Verification items for the finished model (mm, model axes). A direction names the side the tool comes from. Coordinates: 2 decimals unless noted, no trailing zeros. Order: outer loops, then holes, each group sorted by start corner. A loop starts at its lowest first (then second) coordinate and runs counter-clockwise, first axis right, second up. Notation, with made-up numbers: M 1.25,43.25 L 32.25,43.25 A21 cw 32.25,63.25 Z; hole C 87,-36 d1. An arc over 180 degrees is marked long. Write item = value, one per line.
```python
from build123d import *

# Parameters (mm, degrees)
SKETCH1_R           = 100
BOSS_EXTRUDE2_DEPTH = 3
SKETCH5_W           = 3
SKETCH5_H           = 87
BOSS_EXTRUDE5_DEPTH = 45
SKETCH8_W           = 3
SKETCH8_H           = 87
BOSS_EXTRUDE6_DEPTH = 45
SKETCH9_W           = 23.719660605
SKETCH9_H           = 94.301811056
CUT_EXTRUDE2_DEPTH  = 45
SKETCH10_W          = 23.969699351
SKETCH10_H          = 92.447375273
CUT_EXTRUDE3_DEPTH  = 45
SKETCH11_R          = 6
CUT_EXTRUDE4_DEPTH  = 45
SKETCH12_R          = 6
CUT_EXTRUDE5_DEPTH  = 45
BOSS_EXTRUDE7_DEPTH = 45
CUT_EXTRUDE6_DEPTH  = 45


with BuildPart() as part:
    # Sketch1 → Boss-Extrude2 (new body)
    with BuildSketch(Plane(origin=(0, 0, 0), x_dir=(1, 0, 0), z_dir=(0, 1, 0))):
        with Locations(Location((0, 0, 0), (0, 0, 270))):
            Circle(SKETCH1_R)
    extrude(amount=BOSS_EXTRUDE2_DEPTH)

    # Sketch5 → Boss-Extrude5 (add)
    with BuildSketch(Plane(origin=(0, 3, 0), x_dir=(1, 0, 0), z_dir=(0, 1, 0))):
        with Locations((88.5, 0.088989435)):
            Rectangle(SKETCH5_W, SKETCH5_H)
    extrude(amount=BOSS_EXTRUDE5_DEPTH)

    # Sketch8 → Boss-Extrude6 (add)
    with BuildSketch(Plane(origin=(0, 3, 0), x_dir=(1, 0, 0), z_dir=(0, 1, 0))):
        with Locations((-88.5, 0.088989435)):
            Rectangle(SKETCH8_W, SKETCH8_H)
    extrude(amount=BOSS_EXTRUDE6_DEPTH)

    # Sketch9 → Cut-Extrude2 (cut)
    with BuildSketch(Plane(origin=(0, 3, 0), x_dir=(1, 0, 0), z_dir=(0, 1, 0))):
        with Locations((101.859830303, -3.561916093)):
            Rectangle(SKETCH9_W, SKETCH9_H)
    extrude(amount=-CUT_EXTRUDE2_DEPTH, mode=Mode.SUBTRACT)

    # Sketch10 → Cut-Extrude3 (cut)
    with BuildSketch(Plane(origin=(0, 3, 0), x_dir=(1, 0, 0), z_dir=(0, 1, 0))):
        with Locations((-101.984849676, 2.812677071)):
            Rectangle(SKETCH10_W, SKETCH10_H)
    extrude(amount=-CUT_EXTRUDE3_DEPTH, mode=Mode.SUBTRACT)

    # Sketch11 → Cut-Extrude4 (cut)
    with BuildSketch(Plane.ZY.offset(90)):
        with Locations((0, 33)):
            Circle(SKETCH11_R)
    extrude(amount=-CUT_EXTRUDE4_DEPTH, mode=Mode.SUBTRACT)

    # Sketch12 → Cut-Extrude5 (cut)
    with BuildSketch(Plane(origin=(90, 0, 0), x_dir=(0, 0, -1), z_dir=(1, 0, 0))):
        with Locations(Location((0, 33, 0), (0, 0, 180))):
            Circle(SKETCH12_R)
    extrude(amount=-CUT_EXTRUDE5_DEPTH, mode=Mode.SUBTRACT)

    # Sketch14 → Boss-Extrude7 (add)
    with BuildSketch(Plane(origin=(0, 3, 0), x_dir=(1, 0, 0), z_dir=(0, 1, 0))):
        with BuildLine():
            Line((-90, -43.411010565), (-90.085982049, -43.411010565))
            ThreePointArc((-90.085982049, -43.411010565), (-0.098829893, -99.999951163), (90, -43.588989435))
            Line((90, -43.588989435), (90, -43.411010565))
            Line((90, -43.411010565), (87, -43.411010565))
            Line((87, -43.411010565), (87, 43.588989435))
            Line((87, 43.588989435), (90, 43.588989435))
            ThreePointArc((90, 43.588989435), (0, 100), (-90, 43.588989435))
            Line((-90, 43.588989435), (-87, 43.588989435))
            Line((-87, 43.588989435), (-87, -43.411010565))
            Line((-87, -43.411010565), (-90, -43.411010565))
        make_face()
    extrude(amount=BOSS_EXTRUDE7_DEPTH)

    # 3DSketch1 → Cut-Extrude6 (cut)
    with BuildSketch(Plane(origin=(-87, 48, -42.895221179), x_dir=(0.8969072164948455, 0, 0.4422187750417981), z_dir=(0, -1, 0))):
        with BuildLine():
            Line((0, 0), (37.93814433, 76.946066857))
            ThreePointArc((37.93814433, 76.946066857), (139.895221179, 87), (194, 0))
            Line((194, 0), (156.06185567, -76.946066857))
            ThreePointArc((156.06185567, -76.946066857), (54.104778821, -87), (0, 0))
        make_face()
    extrude(amount=CUT_EXTRUDE6_DEPTH, mode=Mode.SUBTRACT)


solid = part.part
```
Item 1: Scan lines: L1, parallel to X at y = 14, z = 41.5; L2, parallel to Y at x = 89, z = 0; L3, parallel to Z at x = -2, y = 7.5. Record each from-to range of solid material in increasing order. Write a range as from..to.
Report:
L1 = -90..-87, 87..90
L2 = 0..27, 39..48
L3 = -99.98..-96.98, 96.98..99.98
Item 2: Sectioned sample at B-B, the plane z = 0. Enter the section's corners in (x, y), then the cut area to 3 significant figures.
Report:
outline = M -90,0 L 90,0 L 90,27 L 87,27 L 87,3 L -87,3 L -87,27 L -90,27 Z; M -90,39 L -87,39 L -87,48 L -90,48 Z; M 87,39 L 90,39 L 90,48 L 87,48 Z
area = 738 mm^2
Item 3: Sectioned sample at A-A, the plane y = 33. Enter the section's corners in (x, z), then the cut area to 3 significant figures.
Report:
outline = M -90.09,43.41 L -90,43.41 L -90,6 L -87,6 L -87,42.9 A97 cw 87,42.9 L 87,6 L 90,6 L 90,43.59 A100 ccw Z; M -90,-43.59 A100 ccw 90,-43.59 L 90,-6 L 87,-6 L 87,-42.9 A97 cw -87,-42.9 L -87,-6 L -90,-6 Z
area = 1,770 mm^2
Item 4: Gauge pin test, flat ends, axial feed: pin 1 (22.5 mm diameter, centred on y = 17.5, z = 4.5, fed in from -X); pin 2 (1 mm diameter, centred on x = -25.5, z = -46.5, fed in from +Y); pin 3 (8 mm diameter, centred on x = 22, y = 38, fed in from +Z). Record the tip position at first contact, or that the pin passes through.
Report:
pin_1 = -90
pin_2 = 3
pin_3 = 98.37
Item 5: Release check for a two-part mould opening along X. For faces 1 (the flat face through (-87, 26, -1)), 2 (the flat face through (-90, 24, 1)), 3 (the flat face through (1, 0, -1)) record: pulls with the +X half, pulls with the -X half, needs draft (parallel to the pull), parting line crosses it, or undercut.
Report:
face_1 = undercut
face_2 = pulls with the -X half
face_3 = needs draft
Item 6: Tool access check on faces 4 (the flat face through (87, 26, 1)), 5 (the cylindrical face through (-88.521, 27.143, -1.301)). Record the directions out of +Z, -Z, +X, -X, +Y, -Y that give a thin tool (end or side, any length) a straight path to the whole face; none if there is none.
Report:
face_4 = +Y
face_5 = +X, -X
Item 7: Sectioned sample at D-D, the plane z = 51. Enter the section's corners in (x, y), then the cut area to 3 significant figures.
Report:
outline = M -86.02,0 L 86.02,0 L 86.02,48 L 82.51,48 L 82.51,3 L -82.51,3 L -82.51,48 L -86.02,48 Z
area = 832 mm^2
Item 8: Sectioned sample at C-C, the plane y = 23. Enter the section's corners in (x, z), then the cut area to 3 significant figures.
Report:
outline = M -90.09,43.41 L -90,43.41 L -90,-43.59 A100 ccw 90,-43.59 L 90,43.59 A100 ccw Z; hole M -87,-42.9 A97 ccw 87,-42.9 L 87,42.9 A97 ccw -87,42.9 Z
area = 1,840 mm^2
